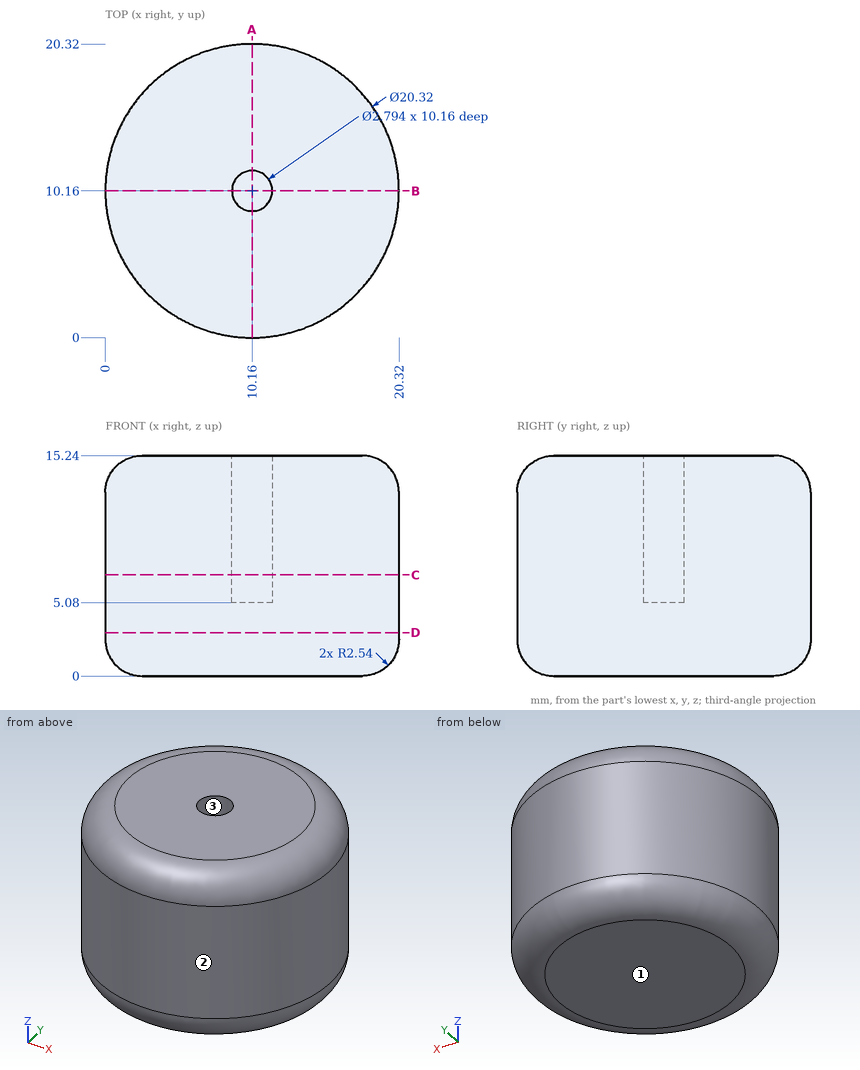
Design review of the part shown in the three views and the two pictorial views. Dimensions are in mm from the part's minimum x, y and z. Give positions to 0.01 mm unless a question says otherwise; leave off trailing zeros. Loops run counter-clockwise (first coordinate to the right, second up) from the corner with the lowest first, then second, coordinate; pieces in that order, holes last. Notation, with made-up numbers: (25.25, 51.25) - (72.25, 51.25) arc R25 ccw to (72.25, 84.25) - close; hole circle Ø4 at (42, 57.5). An arc over 180 degrees is marked (long way). Write item = value, one per line.
1) Take a section at C-C on z = 7. State the section outline as (x, y) points.
Result sheet:
outline = circle Ø20.32 at (10.16, 10.16); hole circle Ø2.79 at (10.16, 10.16)
2) Draft analysis for pull direction X (two halves, no side actions). For the marked faces 1, 2 and 3, state which applies: +X half, -X half, draft (parallel to the pull), parting line (faces both ways), or undercut.
Result sheet:
face_1 = draft
face_2 = parting line
face_3 = undercut
3) To check wall thickness, follow line 1 (Y direction, x = 10.16, z = 12.25); line 2 (Y direction, x = 9, z = 11); line 3 (Y direction, x = 3.5, z = 6.25). State the ranges of each line that lie inside material, in increasing order.
Result sheet:
line_1 = 0 to 8.76, 11.56 to 20.32
line_2 = 0.07 to 9.38, 10.94 to 20.25
line_3 = 2.49 to 17.83
4) Take a section at A-A on x = 10.16. State the section outline as (y, z) points.
Result sheet:
outline = (0, 2.54) arc R2.54 ccw to (2.54, 0) - (17.78, 0) arc R2.54 ccw to (20.32, 2.54) - (20.32, 12.7) arc R2.54 ccw to (17.78, 15.24) - (11.56, 15.24) - (11.56, 5.08) - (8.76, 5.08) - (8.76, 15.24) - (2.54, 15.24) arc R2.54 ccw to (0, 12.7) - close
5) Clearance check with flat-ended pins moving along their axes: pin 1 Ø3 at (y, z) = (15.5, 12.5) entering from -X; pin 2 Ø1 at (y, z) = (13, 9.5) entering from +X; pin 3 Ø1.5 at (x, z) = (12.5, 9) entering from -Y. State where each tip first meets the part, or that it passes through.
Result sheet:
pin_1 = 0.75
pin_2 = 20.05
pin_3 = 0.13
6) Take a section at D-D on z = 3. State the section outline as (x, y) points, and give its area (3 significant figures).
Result sheet:
outline = circle Ø20.32 at (10.16, 10.16)
area = 324 mm2
